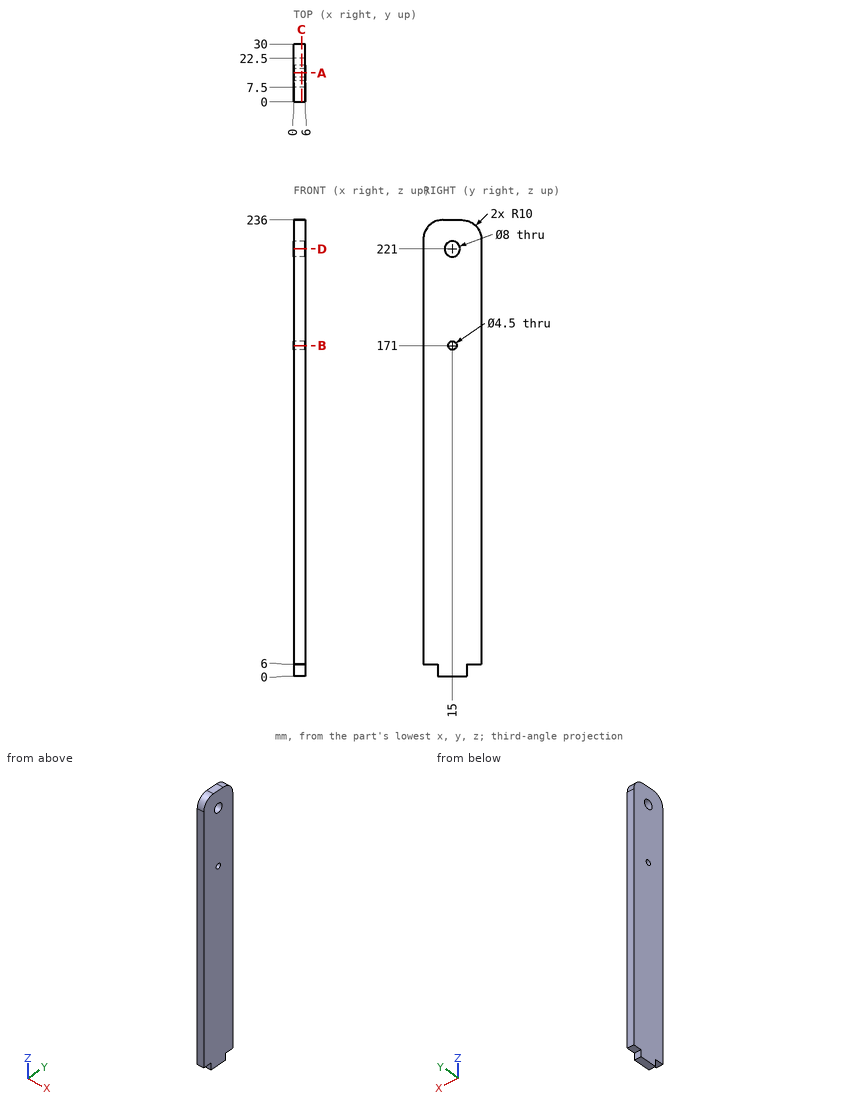
Drawing for the job (mm, zero at the part's lowest x, y, z). Give positions to 0.01 mm unless a question says otherwise; leave off trailing zeros. Order: outer loops, then holes, each group sorted by start corner. A loop starts at its lowest first (then second) coordinate and runs counter-clockwise, first axis right, second up. Notation, with made-up numbers: M -23.5,87.5 L 26.5,87.5 A24 ccw 26.5,100.5 Z; hole C -28.5,-32.75 d2. An arc over 180 degrees is marked long. Put each result on its own line as item: value. Start each with the question number.
(1) Saw through at C-C, the plane x = 4.1. Write the cut outline in (y, z).
(2) Saw through at D-D, the plane z = 221. Write the cut outline in (x, y).
(3) Drill centre lines: line 1 along Y through (x, z) = (3.55, 221); line 2 along Z through (x, y) = (5.55, 9); line 3 along Z through (x, y) = (1.15, 27.5). Where is each one in solid material? Low to high.
(4) Saw through at B-B, the plane z = 171. Write the cut outline in (x, y).
(5) Saw through at A-A, the plane y = 15. Write the cut outline in (x, z).
(6) Flat gauge pins, fed straight in: pin 1 Ø1 at (y, z) = (12.5, 177.5) entering from -X; pin 2 Ø1.8 at (x, z) = (2.5, 1.5) entering from -Y; pin 3 Ø3 at (x, y) = (4, 24.5) entering from -Z. Where does each tip first touch, or does it go through?
Check result:
1. outline: M 0,6 L 7.5,6 L 7.5,0 L 22.5,0 L 22.5,6 L 30,6 L 30,226 A10 ccw 20,236 L 10,236 A10 ccw 0,226 Z; hole C 15,221 d8; hole C 15,171 d4.5
2. outline: M 0,0 L 6,0 L 6,11 L 0,11 Z; M 0,19 L 6,19 L 6,30 L 0,30 Z
3. line 1: y = 0 to 11, 19 to 30
3. line 2: z = 0 to 235.95
3. line 3: z = 6 to 232.61
4. outline: M 0,0 L 6,0 L 6,12.75 L 0,12.75 Z; M 0,17.25 L 6,17.25 L 6,30 L 0,30 Z
5. outline: M 0,0 L 6,0 L 6,168.75 L 0,168.75 Z; M 0,173.25 L 6,173.25 L 6,217 L 0,217 Z; M 0,225 L 6,225 L 6,236 L 0,236 Z
6. pin 1: stops at x = 0
6. pin 2: stops at y = 7.5
6. pin 3: stops at z = 6
